For this review, take the finished solid that the model builds, in its own axes (mm). Face numbers are marked on the shaded views. A direction names the side the tool comes from. Coordinates: 2 decimals unless noted, no trailing zeros. Loops run counter-clockwise (first coordinate to the right, second up) from the corner with the lowest first, then second, coordinate; pieces in that order, holes last. Notation, with made-up numbers: (-38, 14) -> (3, 14) arc R23 ccw to (3, 40) -> close; hole circle Ø10 at (48.25, -40). An arc over 180 degrees is marked (long way). One line per item, written item: value.
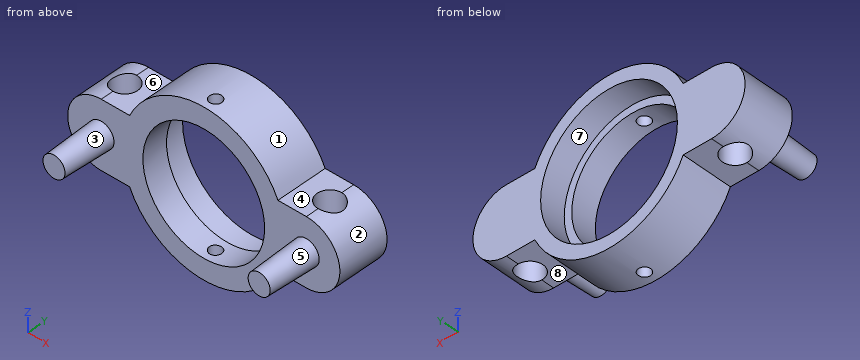
from build123d import *

# Parameters (mm, degrees)
SKETCH1_R                          = 11.303
BOSS_EXTRUDE1_DEPTH                = 9.525
F_4_40_TAPPED_HOLE1_D              = 2.2606
SKETCH10_R                         = 2.38125
BOSS_EXTRUDE2_DEPTH                = 9.525
BOSS_EXTRUDE2_TAPER                = 2
F_3_16_0_1875_DIAMETER_HOLE1_D     = 4.7625
F_3_16_0_1875_DIAMETER_HOLE1_DEPTH = 25.4
F_3_16_0_1875_DIAMETER_HOLE1_TIP   = 1.430799349
SKETCH14_R                         = 12.7
CUT_EXTRUDE1_DEPTH                 = 4.7625


with BuildPart() as part:
    # Sketch1 → Boss-Extrude1 (new body)
    with BuildSketch(Plane(origin=(0, 0, 0), x_dir=(1, 0, 0), z_dir=(0, 1, 0))):
        with BuildLine():
            Line((-19.05, 6.223), (-13.772328779, 6.223))
            ThreePointArc((-13.772328779, 6.223), (0, 15.113), (13.772328779, 6.223))
            Line((13.772328779, 6.223), (19.05, 6.223))
            ThreePointArc((19.05, 6.223), (25.273, 0), (19.05, -6.223))
            Line((19.05, -6.223), (13.772328779, -6.223))
            ThreePointArc((13.772328779, -6.223), (0, -15.113), (-13.772328779, -6.223))
            Line((-13.772328779, -6.223), (-19.05, -6.223))
            ThreePointArc((-19.05, -6.223), (-25.273, 0), (-19.05, 6.223))
        make_face()
        Circle(SKETCH1_R, mode=Mode.SUBTRACT)
    extrude(amount=BOSS_EXTRUDE1_DEPTH)

    # #4-40 Tapped Hole1 (through all)
    with Locations(Plane.XY.offset(15.113)):
        with Locations((0, 2.38125)):
            Hole(F_4_40_TAPPED_HOLE1_D / 2)

    # Sketch10 → Boss-Extrude2 (add)
    with BuildSketch(Plane.XZ):
        with Locations((-19.05, 0)):
            Circle(SKETCH10_R)
        with Locations((19.05, 0)):
            Circle(SKETCH10_R)
    extrude(amount=BOSS_EXTRUDE2_DEPTH, taper=BOSS_EXTRUDE2_TAPER)

    # 3/16 (0.1875) Diameter Hole1
    with Locations(Plane.XY.offset(6.223)):
        with Locations((-19.05, 4.7625), (19.05, 4.7625)):
            Hole(F_3_16_0_1875_DIAMETER_HOLE1_D / 2, depth=F_3_16_0_1875_DIAMETER_HOLE1_DEPTH)
            with Locations((0, 0, -(F_3_16_0_1875_DIAMETER_HOLE1_DEPTH + F_3_16_0_1875_DIAMETER_HOLE1_TIP / 2))):  # 118° drill point
                Cone(0, F_3_16_0_1875_DIAMETER_HOLE1_D / 2, F_3_16_0_1875_DIAMETER_HOLE1_TIP, mode=Mode.SUBTRACT)

    # Sketch14 → Cut-Extrude1 (cut)
    with BuildSketch(Plane(origin=(0, 9.525, 0), x_dir=(1, 0, 0), z_dir=(0, 1, 0))):
        Circle(SKETCH14_R)
    extrude(amount=-CUT_EXTRUDE1_DEPTH, mode=Mode.SUBTRACT)


solid = part.part
1. Take a section at B-B, the plane x = 0. Give the boundary of the cut face in (y, z) (1 decimal).
Return value:
outline: (0, -15.1) -> (1.3, -15.1) -> (1.3, -11.3) -> (0, -11.3) -> close; (0, 11.3) -> (1.3, 11.3) -> (1.3, 15.1) -> (0, 15.1) -> close; (3.5, -15.1) -> (9.5, -15.1) -> (9.5, -12.7) -> (4.8, -12.7) -> (4.8, -11.3) -> (3.5, -11.3) -> close; (3.5, 11.3) -> (4.8, 11.3) -> (4.8, 12.7) -> (9.5, 12.7) -> (9.5, 15.1) -> (3.5, 15.1) -> close
2. Insertion check: pin 1 Ø1 at (x, z) = (-13, 5.5) entering from -Y; pin 2 Ø4 at (x, y) = (-16.5, 5.5) entering from -Z; pin 3 Ø7.5 at (x, y) = (-19.05, 4.76) entering from +Z; pin 4 Ø6 at (x, y) = (12, -5) entering from +Z. Each pin has a flat end and moves straight along its axis. Give the tip position at first contact, or say it passes through.
Return value:
pin 1: stops at y = 0
pin 2: stops at z = -6.22
pin 3: stops at z = 6.22
pin 4: passes through
3. For the marked faces 4, 5, 6, 7 and 8, list the 3-axis set-ups (+Z, -Z, +X, -X, +Y, -Y) from which the entire face can be reached by the end or side of a thin tool; tool diameter is ignored.
Return value:
face 4: +Z, +X, +Y, -Y
face 5: -Y
face 6: +Z, -X, +Y, -Y
face 7: +Y
face 8: -Z, +X, +Y, -Y
4. To check wall thickness, follow probe 1 along X at (y, z) = (5, 0); probe 2 along Z at (x, y) = (0, 3.75); probe 3 along Z at (x, y) = (0, 6.25). State the ranges of each line that lie inside material, in increasing order. Write a range as from..to.
Return value:
probe 1: x = -25.27..-21.42, -16.68..-12.7, 12.7..16.68, 21.42..25.27
probe 2: z = -15.11..-11.3, 11.3..15.11
probe 3: z = -15.11..-12.7, 12.7..15.11
5. Take a section at A-A, the plane z = -4. Give the number of separate pieces and of enclosed holes in the cut face, and give its area (3 significant figures).
Return value:
separate pieces: 2
enclosed holes: 2
area: 203 mm2
6. Take a section at C-C, the plane y = 6.5. Give the boundary of the cut face in (x, z).
Return value:
outline: (-20.68, -6.01) -> (-20.68, 6.01) arc R6.22 ccw to start; (-17.42, -6.22) -> (-13.77, -6.22) arc R15.11 ccw to (13.77, -6.22) -> (17.42, -6.22) -> (17.42, 6.22) -> (13.77, 6.22) arc R15.11 ccw to (-13.77, 6.22) -> (-17.42, 6.22) -> close; (20.68, -6.01) arc R6.22 ccw to (20.68, 6.01) -> close; hole circle Ø25.4 at (0, 0)
7. Take a section at D-D, the plane y = 3. Give the boundary of the cut face in (x, z).
Return value:
outline: (-20.65, -6.01) -> (-20.65, 6.01) arc R6.22 ccw to start; (-17.45, -6.22) -> (-13.77, -6.22) arc R15.11 ccw to (-0.95, -15.08) -> (-0.95, -11.26) arc R11.3 cw to (-0.95, 11.26) -> (-0.95, 15.08) arc R15.11 ccw to (-13.77, 6.22) -> (-17.45, 6.22) -> close; (0.95, -15.08) arc R15.11 ccw to (13.77, -6.22) -> (17.45, -6.22) -> (17.45, 6.22) -> (13.77, 6.22) arc R15.11 ccw to (0.95, 15.08) -> (0.95, 11.26) arc R11.3 cw to (0.95, -11.26) -> close; (20.65, -6.01) arc R6.22 ccw to (20.65, 6.01) -> close
8. The part is to be moulded in two halves that separate along X. For the marked faces 1, 2 and 3, say which applies: pulls with the +X half, pulls with the -X half, needs draft (parallel to the pull), parting line crosses it, or undercut.
Return value:
face 1: parting line crosses it
face 2: pulls with the +X half
face 3: undercut
